```python
from build123d import *

# Parameters (mm, degrees)
F0_W     = 36
F0_H     = 36
F1_DEPTH = 36
F2_R     = 16
F2_R_2   = 15.8
F3_DEPTH = 2
F4_R     = 1.25
F5_DEPTH = 36.001
F6_R     = 1.25
F7_DEPTH = 36.001
F8_SIZE  = 4


with BuildPart() as f1:
    # F0 (on Front) → F1 (new body)
    with BuildSketch(Plane.XZ):
        Rectangle(F0_W, F0_H)
    extrude(amount=F1_DEPTH)

    # F2 (on face) → F3 (cut)
    with BuildSketch(Plane.XZ.offset(36)):
        Circle(F2_R)
        Circle(F2_R_2, mode=Mode.SUBTRACT)
    extrude(amount=-F3_DEPTH, mode=Mode.SUBTRACT)

    # F4 (on face) → F5 (cut, through all)
    with BuildSketch(Plane.YZ.offset(18)):
        with Locations((-30, 12)):
            Circle(F4_R)
        with Locations((-6, 12)):
            Circle(F4_R)
        with Locations((-6, -12)):
            Circle(F4_R)
        with Locations((-30, -12)):
            Circle(F4_R)
    extrude(amount=-F5_DEPTH, mode=Mode.SUBTRACT)

    # F6 (on face) → F7 (cut, through all)
    with BuildSketch(Plane.XY.offset(18)):
        with Locations((-12, -30)):
            Circle(F6_R)
        with Locations((-12, -6)):
            Circle(F6_R)
        with Locations((12, -6)):
            Circle(F6_R)
        with Locations((12, -30)):
            Circle(F6_R)
    extrude(amount=-F7_DEPTH, mode=Mode.SUBTRACT)

    # F8
    f8_edges = [f1.edges().sort_by_distance(p)[0] for p in [
        (18, -18, 18),
        (-18, -18, 18),
        (18, -18, -18),
        (-18, -18, -18),
    ]]
    chamfer(f8_edges, length=F8_SIZE)


solid = f1.part
```
Model file for the job. Use its own axes, mm. A direction names the side the tool comes from. Coordinates: 2 decimals unless noted, no trailing zeros. Loops run counter-clockwise (first coordinate to the right, second up) from the corner with the lowest first, then second, coordinate; pieces in that order, holes last. Notation, with made-up numbers: (0, -6.5) - (23, -6.5) arc R30 ccw to (23, 23.5) - close; hole circle Ø10 at (-32, 88.5). An arc over 180 degrees is marked (long way). Write item = value, one per line. Start each with the question number.
Item 1: Pull direction Y, two halves, no side cores. Call faces 3 (the face through (-16, -18, 16)), 4 (the face through (11.079, -5.155, -15.625)), 5 (the face through (0, 0, 0)): +Y half, -Y half, draft (parallel to the pull), parting line (faces both ways), or undercut.
Item 2: Drop a flat-ended pin along its axis: pin 1 Ø2 at (x, y) = (-12, -6) entering from -Z. Give the stop position or say it passes through.
Item 3: 3-axis set-ups, long thin cutter, end or side, ignore diameter. For faces 1 (the face through (-12.54, -35.01, -9.61)), 2 (the face through (-16.3, -36, 0.3)): which of +Z, -Z, +X, -X, +Y, -Y reach the whole face in a straight line?
Item 4: Saw through at A-A, the plane z = 0. List the corners of the cut face in (x, y), then the cut area to 3 significant figures.
Item 5: Saw through at D-D, the plane y = -6. State how many separate pieces and enclosed holes the cut face has, then the cut area to 3 significant figures.
Item 6: Saw through at C-C, the plane y = -25.5. List the corners of the cut face in (x, z).
Item 7: Saw through at B-B, the plane x = 0. List the corners of the cut face in (y, z), then the cut area to 3 significant figures.
Item 8: Wall check: probe 1 along Y at (x, z) = (-12, 16.65); probe 2 along Z at (x, y) = (-4.5, -30); probe 3 along Z at (x, y) = (0, -35.1). Give the ranges that are in metal, low to high. Write a range as [from, to].
Answers:
q1.face_3 = draft
q1.face_4 = undercut
q1.face_5 = +Y half
q2.pin_1 = through
q3.face_1 = -Y
q3.face_2 = +Z, -Z, +X, -X, -Y
q4.outline = (-18, -36) - (-16, -36) - (-16, -34) - (-15.8, -34) - (-15.8, -36) - (15.8, -36) - (15.8, -34) - (16, -34) - (16, -36) - (18, -36) - (18, 0) - (-18, 0) - close; hole circle Ø2.5 at (-12, -30); hole circle Ø2.5 at (-12, -6); hole circle Ø2.5 at (12, -30); hole circle Ø2.5 at (12, -6)
q4.area = 1,280 mm2
q5.separate_pieces = 9
q5.enclosed_holes = 0
q5.area = 929 mm2
q6.outline = (-18, -14) - (-14, -18) - (14, -18) - (18, -14) - (18, 14) - (14, 18) - (-14, 18) - (-18, 14) - close
q7.outline = (-36, -18) - (0, -18) - (0, 18) - (-36, 18) - (-36, 16) - (-34, 16) - (-34, 15.8) - (-36, 15.8) - (-36, -15.8) - (-34, -15.8) - (-34, -16) - (-36, -16) - close; hole circle Ø2.5 at (-30, -12); hole circle Ø2.5 at (-30, 12); hole circle Ø2.5 at (-6, -12); hole circle Ø2.5 at (-6, 12)
q7.area = 1,280 mm2
q8.probe_1 = [-36, -31.25], [-28.75, -7.25], [-4.75, 0]
q8.probe_2 = [-18, -13.25], [-10.75, 10.75], [13.25, 18]
q8.probe_3 = [-18, -16], [-15.8, 15.8], [16, 18]
